```python
from build123d import *

# Parameters (mm, degrees)
SKETCH1_W           = 9
SKETCH1_H           = 2.3
BOSS_EXTRUDE1_DEPTH = 15
CUT_EXTRUDE1_START  = -31
SKETCH2_W           = 8
SKETCH2_H           = 0.5
CUT_EXTRUDE1_DEPTH  = 32


with BuildPart() as part:
    # Sketch1 → Boss-Extrude1 (new body, symmetric)
    with BuildSketch(Plane(origin=(0, 0, 0), x_dir=(1, 0, 0), z_dir=(0, 1, 0))):
        Rectangle(SKETCH1_W, SKETCH1_H)
    extrude(amount=BOSS_EXTRUDE1_DEPTH, both=True)

    # Sketch2 → Cut-Extrude1 (cut)
    with BuildSketch(Plane(origin=(0, 15, 0), x_dir=(1, 0, 0), z_dir=(0, 1, 0)).offset(CUT_EXTRUDE1_START)):
        with Locations((0, 0.5)):
            Rectangle(SKETCH2_W, SKETCH2_H)
    cut_extrude1 = extrude(amount=CUT_EXTRUDE1_DEPTH, mode=Mode.SUBTRACT)

    # Mirror1: Cut-Extrude1 across plane
    add(cut_extrude1.mirror(Plane.XY), mode=Mode.SUBTRACT)


solid = part.part
```
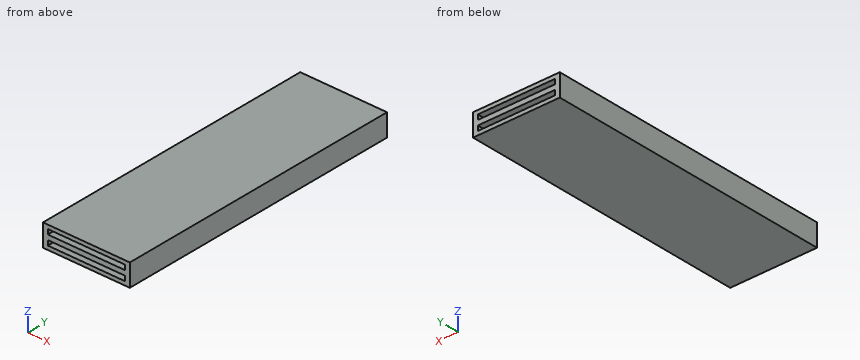
Design review of the part built by this model. Coordinates are the model's own, in mm. Coordinates: 2 decimals unless noted, no trailing zeros. Loops run counter-clockwise (first coordinate to the right, second up) from the corner with the lowest first, then second, coordinate; pieces in that order, holes last. Notation, with made-up numbers: (60.5, 22) -> (111.5, 22) arc R34 ccw to (111.5, 61) -> close; hole circle Ø2 at (-12, 55.25). An arc over 180 degrees is marked (long way). Answer as a JSON object with one key per item and string values.
Q1. Take a section at B-B on y = -10.25. Give the boundary of the cut face in (x, z).
Answer block:
{"outline": "(-4.5, -1.15) -> (4.5, -1.15) -> (4.5, 1.15) -> (-4.5, 1.15) -> close; hole (-4, -0.75) -> (4, -0.75) -> (4, -0.25) -> (-4, -0.25) -> close; hole (-4, 0.25) -> (4, 0.25) -> (4, 0.75) -> (-4, 0.75) -> close"}
Q2. Take a section at A-A on x = -0.5. Give the boundary of the cut face in (y, z), plus the area to 3 significant figures.
Answer block:
{"outline": "(-15, -1.15) -> (15, -1.15) -> (15, -0.75) -> (-15, -0.75) -> close; (-15, -0.25) -> (15, -0.25) -> (15, 0.25) -> (-15, 0.25) -> close; (-15, 0.75) -> (15, 0.75) -> (15, 1.15) -> (-15, 1.15) -> close", "area": "39.0 mm^2"}
Q3. To check wall thickness, follow L1, parallel to Z at x = -0.75, y = -7.5; L2, parallel to X at y = 1.5, z = 0.5. State the ranges of each line that lie inside material, in increasing order.
Answer block:
{"L1": "z = -1.15 to -0.75, -0.25 to 0.25, 0.75 to 1.15", "L2": "x = -4.5 to -4, 4 to 4.5"}
